from build123d import *

# Parameters (mm, degrees)
SKETCH1_R           = 1.5
SKETCH1_R_2         = 1.25
BOSS_EXTRUDE1_DEPTH = 2.5


with BuildPart() as part:
    # Sketch1 → Boss-Extrude1 (new body)
    with BuildSketch(Plane(origin=(0, 0, 0), x_dir=(0, 0, -1), z_dir=(1, 0, 0))):
        with BuildLine():
            Line((-7, 0), (-7, 53.695339599))
            Line((-7, 53.695339599), (7, 53.695339599))
            Line((7, 53.695339599), (7, 0))
            ThreePointArc((7, 0), (0, -7), (-7, 0))
        make_face()
        Circle(SKETCH1_R, mode=Mode.SUBTRACT)
        with Locations((0, 45)):
            Circle(SKETCH1_R_2, mode=Mode.SUBTRACT)
        with Locations((0, 40)):
            Circle(SKETCH1_R_2, mode=Mode.SUBTRACT)
        with Locations((0, 35)):
            Circle(SKETCH1_R_2, mode=Mode.SUBTRACT)
        with Locations((0, 30)):
            Circle(SKETCH1_R_2, mode=Mode.SUBTRACT)
    extrude(amount=BOSS_EXTRUDE1_DEPTH)


solid = part.part
The model under review builds one solid part; all positions refer to its coordinate system, in mm. Give positions to 0.01 mm unless a question says otherwise; leave off trailing zeros. Order: outer loops, then holes, each group sorted by start corner. A loop starts at its lowest first (then second) coordinate and runs counter-clockwise, first axis right, second up. Notation, with made-up numbers: (33.5, 37.25) -> (77.5, 37.25) arc R12 cw to (77.5, 46.25) -> close; hole circle Ø8 at (-37, 50.5). An arc over 180 degrees is marked (long way). Write item = value, one per line. Start each with the question number.
(1) Take a section at C-C (y = 0.5). Write out the cut boundary in (x, z).
(2) Take a section at D-D (z = -3.5). Write out the cut boundary in (x, y).
(3) Take a section at B-B (x = 1). Write out the cut boundary in (y, z), plus the area to 3 significant figures.
(4) Draft analysis for pull direction Y (two halves, no side actions). For faces 1 (the cylindrical face through (1.23, 46.24, 0.16)), 2 (the flat face through (1, 26, 7)), 3 (the cylindrical face through (1.23, 28.78, 0.27)), 4 (the flat face through (1, 53.695, 0)), state which applies: +Y half, -Y half, draft (parallel to the pull), parting line (faces both ways), or undercut.
(5) For L1, parallel to Y at x = 0.15, z = 0; L2, parallel to Y at x = 2.2, z = 1; L3, parallel to Z at x = 0.8, y = 30.5, list the stretches that pass through material, from the lowest coordinate up. Write a range as from..to.
(6) Take a section at A-A (y = 30). Write out the cut boundary in (x, z).
Returned:
q1.outline = (0, -7) -> (2.5, -7) -> (2.5, -1.41) -> (0, -1.41) -> close; (0, 1.41) -> (2.5, 1.41) -> (2.5, 7) -> (0, 7) -> close
q2.outline = (0, -6.06) -> (2.5, -6.06) -> (2.5, 53.7) -> (0, 53.7) -> close
q3.outline = (0, -7) -> (53.7, -7) -> (53.7, 7) -> (0, 7) arc R7 ccw to start; hole circle Ø3 at (0, 0); hole circle Ø2.5 at (30, 0); hole circle Ø2.5 at (35, 0); hole circle Ø2.5 at (40, 0); hole circle Ø2.5 at (45, 0)
q3.area = 802 mm²
q4.face_1 = undercut
q4.face_2 = draft
q4.face_3 = undercut
q4.face_4 = +Y half
q5.L1 = -7..-1.5, 1.5..28.75, 31.25..33.75, 36.25..38.75, 41.25..43.75, 46.25..53.7
q5.L2 = -6.93..-1.12, 1.12..29.25, 30.75..34.25, 35.75..39.25, 40.75..44.25, 45.75..53.7
q5.L3 = -7..-1.15, 1.15..7
q6.outline = (0, -7) -> (2.5, -7) -> (2.5, -1.25) -> (0, -1.25) -> close; (0, 1.25) -> (2.5, 1.25) -> (2.5, 7) -> (0, 7) -> close
